Answer from the drawing. Dimensions are ordinates in mm from the lowest x, y and z of the part. A direction names the side the tool comes from. Round coordinates to 2 decimals unless told otherwise and drop trailing zeros. Order: outer loops, then holes, each group sorted by start corner. A loop starts at its lowest first (then second) coordinate and runs counter-clockwise, first axis right, second up. Notation, with made-up numbers: (42, 85) -> (55, 85) arc R13 ccw to (55, 106) -> close; hole circle Ø5 at (-23, 35.25). An arc over 180 degrees is marked (long way). Use a Markdown table: item, result. Add a question column.
Item 1: A cutting plane is placed at A-A, the plane y = 39. Determine the outline of the cut face in (x, z), plus the area to 3 significant figures.
Item 2: A flat-ended cylindrical pin translates along its axis: P1, Ø1, axis at x = 305.5, z = 135, coming from the -Y side. Find the tip coordinate at first contact, or state that the pin passes through.
Item 3: For a pull along X with two mould halves and no side action, classify the marked faces 1, 2 and 3 as +X half, -X half, draft (parallel to the pull), parting line (faces both ways), or undercut.
Item 4: A cutting plane is placed at C-C, the plane x = 365. Determine the outline of the cut face in (y, z).
Item 5: A cutting plane is placed at B-B, the plane z = 62. Determine the outline of the cut face in (x, y).
Item 6: Find the intervals of material crossed by L1, parallel to Z at x = 404, y = 26.5; L2, parallel to X at y = 22, z = 39.5; L3, parallel to Y at x = 24, z = 25.5, in increasing order. Write a range as [from, to].
Item 7: A tool of negligible diameter and unlimited length cuts with its end or side. For the marked faces 4 and 5, from which of +Z, -Z, +X, -X, +Y, -Y can it reach the whole face along a straight path? Write none if from no direction.
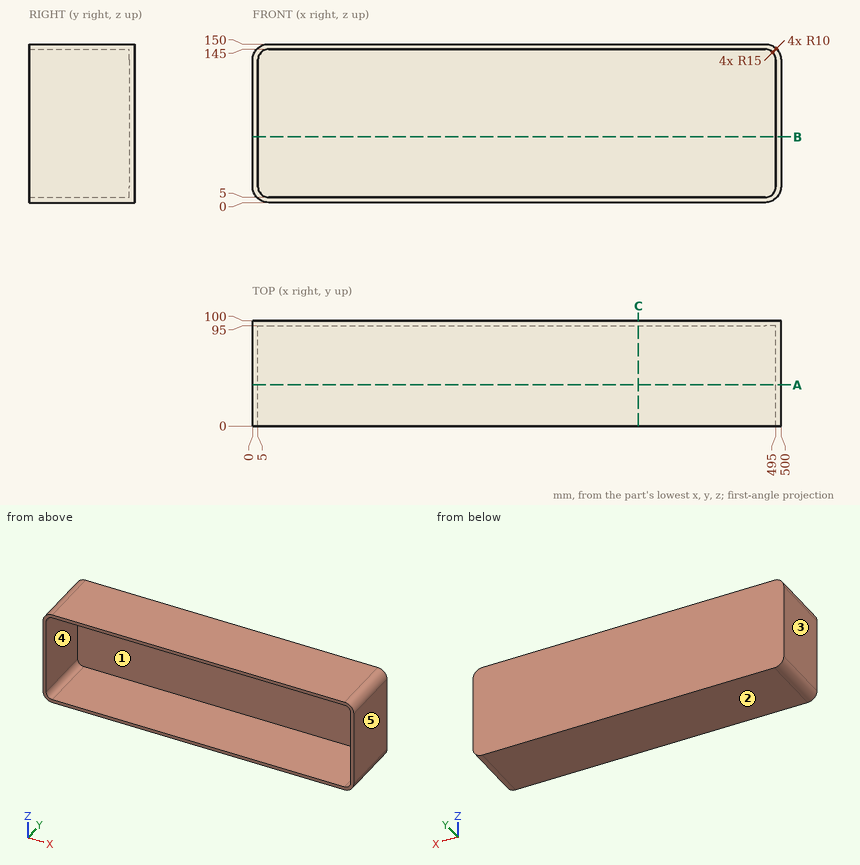
Reported:
| question | item | result |
|---|---|---|
| 1 | outline | (0, 15) arc R15 ccw to (15, 0) -> (485, 0) arc R15 ccw to (500, 15) -> (500, 135) arc R15 ccw to (485, 150) -> (15, 150) arc R15 ccw to (0, 135) -> close; hole (5, 15) arc R10 ccw to (15, 5) -> (485, 5) arc R10 ccw to (495, 15) -> (495, 135) arc R10 ccw to (485, 145) -> (15, 145) arc R10 ccw to (5, 135) -> close |
| 1 | area | 6,290 mm² |
| 2 | P1 | y = 95 |
| 3 | face 1 | undercut |
| 3 | face 2 | draft |
| 3 | face 3 | -X half |
| 4 | outline | (0, 0) -> (100, 0) -> (100, 150) -> (0, 150) -> (0, 145) -> (95, 145) -> (95, 5) -> (0, 5) -> close |
| 5 | outline | (0, 0) -> (5, 0) -> (5, 95) -> (495, 95) -> (495, 0) -> (500, 0) -> (500, 100) -> (0, 100) -> close |
| 6 | L1 | [0, 5], [145, 150] |
| 6 | L2 | [0, 5], [495, 500] |
| 6 | L3 | [95, 100] |
| 7 | face 4 | -Y |
| 7 | face 5 | +Z, -Z, +X, +Y, -Y |
